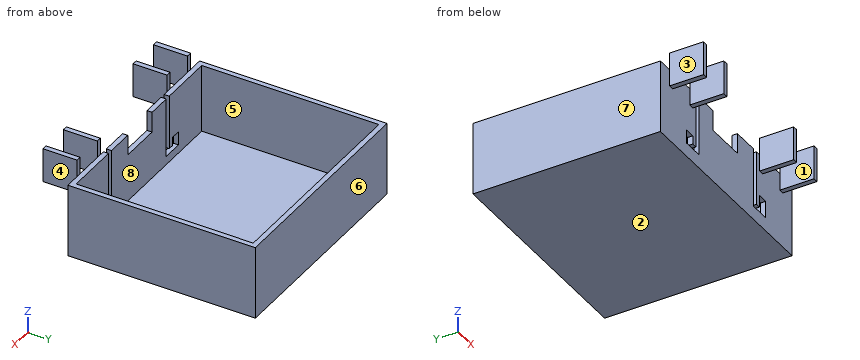
from build123d import *

# Parameters (mm, degrees)
SKETCH_1_W          = 65
SKETCH_1_H          = 55
EXTRUDE_1_DEPTH     = 1.5
SKETCH_2_W          = 65
SKETCH_2_H          = 55
SKETCH_2_W_2        = 62
SKETCH_2_H_2        = 52
EXTRUDE_2_DEPTH     = 20
SKETCH_3_W          = 12
SKETCH_3_H          = 6
CUT_EXTRUDE_1_DEPTH = 1.5
CUT_EXTRUDE_2_DEPTH = 1.5
SKETCH_5_W          = 1.5
SKETCH_5_H          = 10
EXTRUDE_3_DEPTH     = 10


with BuildPart() as part:
    # 草图1 → 凸台-拉伸1 (new body)
    with BuildSketch(Plane.XY):
        with Locations((32.5, -27.5)):
            Rectangle(SKETCH_1_W, SKETCH_1_H)
    extrude(amount=EXTRUDE_1_DEPTH)

    # 草图2 → 凸台-拉伸2 (add)
    with BuildSketch(Plane.XY.offset(1.5)):
        with Locations((32.5, -27.5)):
            Rectangle(SKETCH_2_W, SKETCH_2_H)
        with Locations((32.5, -27.5)):
            Rectangle(SKETCH_2_W_2, SKETCH_2_H_2, mode=Mode.SUBTRACT)
    extrude(amount=EXTRUDE_2_DEPTH)

    # 草图3 → 切除-拉伸1 (cut)
    with BuildSketch(Plane.XZ.offset(55)):
        with Locations((32, 18.5)):
            Rectangle(SKETCH_3_W, SKETCH_3_H)
    extrude(amount=-CUT_EXTRUDE_1_DEPTH, mode=Mode.SUBTRACT)

    # 草图4 → 切除-拉伸2 (cut)
    with BuildSketch(Plane.XZ.offset(55)):
        Polygon((19, 21.5), (17.5, 21.5), (17.5, 5.5), (16, 5.5), (16, 8), (13, 8), (13, 4), (19, 4), align=None)
        Polygon((47.5, 5.5), (47.5, 21.5), (46, 21.5), (46, 4), (52, 4), (52, 9), (49, 9), (49, 5.5), align=None)
    extrude(amount=-CUT_EXTRUDE_2_DEPTH, mode=Mode.SUBTRACT)

    # 草图5 → 凸台-拉伸3 (add)
    with BuildSketch(Plane.XZ.offset(55)):
        with Locations((15.25, 21.5)):
            Rectangle(SKETCH_5_W, SKETCH_5_H)
        with Locations((5.25, 21.5)):
            Rectangle(SKETCH_5_W, SKETCH_5_H)
        with Locations((49.75, 21.5)):
            Rectangle(SKETCH_5_W, SKETCH_5_H)
        with Locations((59.75, 21.5)):
            Rectangle(SKETCH_5_W, SKETCH_5_H)
    extrude(amount=EXTRUDE_3_DEPTH)


solid = part.part
Build history of the part. All positions in model axes, mm. Face numbers are marked on the shaded views. A direction names the side the tool comes from. Round coordinates to 2 decimals unless told otherwise and drop trailing zeros. Write each loop counter-clockwise with the first axis right and the second up, starting at its lowest first coordinate (ties: lowest second). Pieces come first, ordered by that corner, then holes. Notation, with made-up numbers: (56.5, -9.75) -> (93.5, -9.75) arc R8 cw to (93.5, 1.25) -> close; hole circle Ø9 at (-29.5, 68.5). An arc over 180 degrees is marked (long way). Use one line per item in the form item = value.
Q1. Drill centre lines: L1, parallel to X at y = -42, z = 4.5; L2, parallel to Y at x = 25, z = 10.25; L3, parallel to Z at x = 3, y = -32.5. Where is each one in solid material? Low to high.
Conclusion:
L1 = 0 to 1.5, 63.5 to 65
L2 = -55 to -53.5, -1.5 to 0
L3 = 0 to 1.5
Q2. Band-saw the part on C-C, the plane z = 10.25. Write the cut outline in (x, y), then the cut area to 4 significant figures.
Conclusion:
outline = (0, -55) -> (17.5, -55) -> (17.5, -53.5) -> (1.5, -53.5) -> (1.5, -1.5) -> (63.5, -1.5) -> (63.5, -53.5) -> (47.5, -53.5) -> (47.5, -55) -> (65, -55) -> (65, 0) -> (0, 0) -> close; (19, -55) -> (46, -55) -> (46, -53.5) -> (19, -53.5) -> close
area = 346.5 mm²
Q3. Drop flat-ended pins along their axis: P1, Ø5, axis at x = 9.5, z = 19, coming from the -Y side; P2, Ø5, axis at x = 20.5, y = -49, coming from the +Z side; P3, Ø11, axis at y = -61, z = 21, coming from the +X side. Give the stop position or say it passes through.
Conclusion:
P1 = -55
P2 = 1.5
P3 = 60.5
Q4. Band-saw the part on A-A, the plane z = 23. Write the cut outline in (x, y).
Conclusion:
outline = (4.5, -65) -> (6, -65) -> (6, -55) -> (4.5, -55) -> close; (14.5, -65) -> (16, -65) -> (16, -55) -> (14.5, -55) -> close; (49, -65) -> (50.5, -65) -> (50.5, -55) -> (49, -55) -> close; (59, -65) -> (60.5, -65) -> (60.5, -55) -> (59, -55) -> close
Q5. Band-saw the part on B-B, the plane y = -44. Write the cut outline in (x, z).
Conclusion:
outline = (0, 0) -> (65, 0) -> (65, 21.5) -> (63.5, 21.5) -> (63.5, 1.5) -> (1.5, 1.5) -> (1.5, 21.5) -> (0, 21.5) -> close
Q6. Two-plate mould, pull along X, no slides. Class the marked faces 6, 7 and 8: released by +X, released by -X, zero draft, split by the parting line, or undercut.
Conclusion:
face_6 = zero draft
face_7 = released by -X
face_8 = undercut
Q7. Tool access for the marked faces 1, 2, 3, 4 and 5: list every direction of +Z, -Z, +X, -X, +Y, -Y with a clear straight run to the whole face (end or side of a thin tool).
Conclusion:
face_1 = +Z, -Z, -Y
face_2 = -Z, +X, -X, +Y, -Y
face_3 = +Z, -Z, -X, -Y
face_4 = +Z, -Z, +X, -Y
face_5 = +Z
Q8. Band-saw the part on D-D, the plane x = 43.5. Write the cut outline in (y, z), then the cut area to 4 significant figures.
Conclusion:
outline = (-55, 0) -> (0, 0) -> (0, 21.5) -> (-1.5, 21.5) -> (-1.5, 1.5) -> (-53.5, 1.5) -> (-53.5, 21.5) -> (-55, 21.5) -> close
area = 142.5 mm²
